Could you check a few things on this model? Use its own coordinates, in mm. Coordinates: 2 decimals unless noted, no trailing zeros. Loops run counter-clockwise (first coordinate to the right, second up) from the corner with the lowest first, then second, coordinate; pieces in that order, holes last. Notation, with made-up numbers: (-37.75, 64) - (-14.75, 64) arc R31 ccw to (-14.75, 91) - close; hole circle Ø2 at (79.25, 26). An arc over 180 degrees is marked (long way). Use CSV: the item, a comma, the result in double quotes.
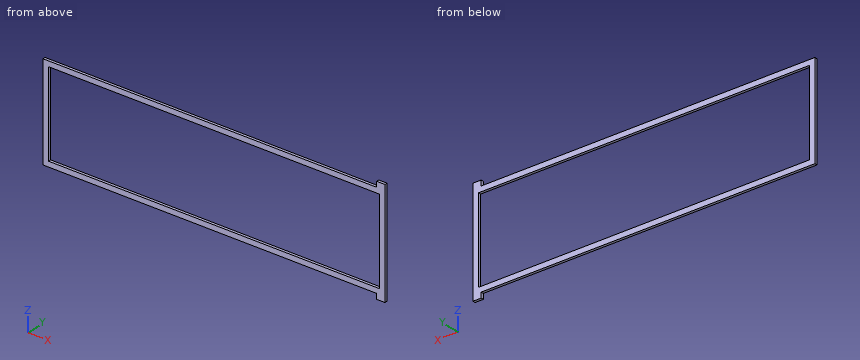
from build123d import *

# Parameters (mm, degrees)
SKETCH1_W           = 393.7
SKETCH1_H           = 101.6508
BOSS_EXTRUDE1_DEPTH = 3.175
SKETCH2_W           = 393.4968
SKETCH2_H           = 101.4476
BOSS_EXTRUDE2_DEPTH = 3.175


with BuildPart() as part:
    # Sketch1 → Boss-Extrude1 (new body)
    with BuildSketch(Plane(origin=(0, 0, 0), x_dir=(1, 0, 0), z_dir=(0, 1, 0))):
        Polygon((193.675, -56.848375), (193.675, -63.223775), (203.2, -63.223775), (203.2, 63.223775), (193.675, 63.223775), (193.675, 56.848375), (-203.2, 56.848375), (-203.2, -56.848375), align=None)
        with Locations((0, -0.0254)):
            Rectangle(SKETCH1_W, SKETCH1_H, mode=Mode.SUBTRACT)
    extrude(amount=BOSS_EXTRUDE1_DEPTH)

    # Sketch2 → Boss-Extrude2 (add)
    with BuildSketch(Plane(origin=(0, 3.175, 0), x_dir=(1, 0, 0), z_dir=(0, 1, 0))):
        Polygon((193.5734, -56.949975), (193.5734, -63.325375), (203.3016, -63.325375), (203.3016, 63.325375), (193.5734, 63.325375), (193.5734, 56.949975), (-203.3016, 56.949975), (-203.3016, -56.949975), align=None)
        with Locations((0, -0.0254)):
            Rectangle(SKETCH2_W, SKETCH2_H, mode=Mode.SUBTRACT)
    extrude(amount=-BOSS_EXTRUDE2_DEPTH)


solid = part.part
(1) Suppose I cut it at A-A (x = -13). Write out the boundary of the cut face in (y, z) (3 decimals).
Computed:
outline,"(0, -56.95) - (3.175, -56.95) - (3.175, -50.698) - (0, -50.698) - close; (0, 50.749) - (3.175, 50.749) - (3.175, 56.95) - (0, 56.95) - close"
(2) Suppose I cut it at B-B (y = 2.6). Write out the boundary of the cut face in (x, z).
Computed:
outline,"(-203.3, -56.95) - (193.57, -56.95) - (193.57, -63.33) - (203.3, -63.33) - (203.3, 63.33) - (193.57, 63.33) - (193.57, 56.95) - (-203.3, 56.95) - close; hole (-196.75, -50.7) - (196.75, -50.7) - (196.75, 50.75) - (-196.75, 50.75) - close"
(3) Will these pins go through, and if not, where does the flat tip stop? pin 1 (1 mm diameter, centred on y = 1, z = 61, fed in from -X); pin 2 (1 mm diameter, centred on x = 32, y = 2, fed in from +Z).
Computed:
pin 1,"stops at x = 193.57"
pin 2,"stops at z = 56.95"
(4) Please list where these lines run through material, in increasing order: line 1 (X direction, y = 2.55, z = -32.5); line 2 (Z direction, x = -47, y = 3.05).
Computed:
line 1,"x = -203.3 to -196.75, 196.75 to 203.3"
line 2,"z = -56.95 to -50.7, 50.75 to 56.95"
(5) Suppose I cut it at C-C (z = 45). Write out the boundary of the cut face in (x, y) (3 decimals).
Computed:
outline,"(-203.302, 0) - (-196.748, 0) - (-196.748, 3.175) - (-203.302, 3.175) - close; (196.748, 0) - (203.302, 0) - (203.302, 3.175) - (196.748, 3.175) - close"
